Part model, mm, in its own coordinate system. A direction names the side the tool comes from. Round coordinates to 2 decimals unless told otherwise and drop trailing zeros. Order: outer loops, then holes, each group sorted by start corner. A loop starts at its lowest first (then second) coordinate and runs counter-clockwise, first axis right, second up. Notation, with made-up numbers: (-26.75, 14.5) - (-9.75, 14.5) arc R25 ccw to (-9.75, 49.5) - close; hole circle Ø4 at (11, -10). An arc over 180 degrees is marked (long way). Return JSON: item names as keys, results as strings. Group by question number.
Item 1: Two-plate mould, pull along Y, no slides. Class faces 4 (the face through (1.174, -2.072, 4.472)), 5 (the face through (-2.381, 0, 4)), 6 (the face through (-0.61, 4.66, 3.14)), 7 (the face through (-3, -2, 0)): released by +Y, released by -Y, zero draft, split by the parting line, or undercut.
Item 2: Drop flat-ended pins along their axis: pin 1 (3 mm diameter, centred on x = 2, y = -3.5, fed in from -Z); pin 2 (5 mm diameter, centred on x = 0, z = -4, fed in from +Y); pin 3 (3 mm diameter, centred on y = -1.5, z = -9, fed in from +X). Give the stop position or say it passes through.
Item 3: Probe probe 1 along Z at (x, y) = (-1.75, 3.25); probe 2 along X at (y, z) = (0.25, 4); probe 3 along Z at (x, y) = (-0.5, 2). List the from-to ranges inside material, lowest first.
Item 4: Saw through at A-A on z = -8. List the corners of the cut face in (x, y).
Item 5: Tool access for faces 1 (the face through (-1.174, 2.072, 4.472)), 2 (the face through (0, 0, -19.05)), 3 (the face through (0.67, -3.04, -9)): list every direction of +Z, -Z, +X, -X, +Y, -Y with a clear straight run to the whole face (end or side of a thin tool).
```python
from build123d import *

# Parameters (mm, degrees)
SKETCH1_W      = 4.699
SKETCH1_H      = 6.35
SKETCH2_R      = 3.1115
EXTRUDE1_DEPTH = 19.05
EXTRUDE2_DEPTH = 3.81
CHAMFER1_SIZE2 = 0.793750001
CHAMFER1_SIZE  = 0.793749999
FILLET1_R      = 0.381
FILLET2_R      = 0.381


with BuildPart() as part:
    # Sketch1 → Revolve1 (revolve)
    with BuildSketch(Plane(origin=(0, 0, 0), x_dir=(1, 0, 0), z_dir=(0, 1, 0))):
        with Locations((2.3495, -3.175)):
            Rectangle(SKETCH1_W, SKETCH1_H)
    revolve(axis=Axis((0, 0, 0), (0, 0, 1)))

    # Sketch2 → Extrude1 (add)
    with BuildSketch(Plane(origin=(0, 0, 0), x_dir=(-1, 0, 0), z_dir=(0, 0, -1))):
        Circle(SKETCH2_R)
    extrude(amount=EXTRUDE1_DEPTH)

    # Sketch3 → Extrude2 (cut)
    with BuildSketch(Plane.XY.offset(6.35)):
        Polygon((2.38125, 1.374815329), (0, 2.749630657), (-2.38125, 1.374815329), (-2.38125, -1.374815329), (0, -2.749630657), (2.38125, -1.374815329), align=None)
    extrude(amount=-EXTRUDE2_DEPTH, mode=Mode.SUBTRACT)

    # Chamfer1
    chamfer1_edges = [part.edges().sort_by_distance(p)[0] for p in [
        (3.1115, 0, -19.05),
    ]]
    chamfer(chamfer1_edges, length=CHAMFER1_SIZE, length2=CHAMFER1_SIZE2)

    # Fillet1
    fillet1_edges = [part.edges().sort_by_distance(p)[0] for p in [
        (-4.699, 0, 6.35),
    ]]
    fillet(fillet1_edges, radius=FILLET1_R)

    # Fillet2
    fillet2_edges = [part.edges().sort_by_distance(p)[0] for p in [
        (-4.699, 0, 0),
    ]]
    fillet(fillet2_edges, radius=FILLET2_R)


solid = part.part
```
Filled in:
{
 "1": {"face 4": "undercut", "face 5": "undercut", "face 6": "split by the parting line", "face 7": "zero draft"},
 "2": {"pin 1": "stops at z = -18.84", "pin 2": "stops at y = 3.11", "pin 3": "stops at x = 3.11"},
 "3": {"probe 1": "z = 0 to 6.35", "probe 2": "x = -4.69 to -2.38, 2.38 to 4.69", "probe 3": "z = -19.05 to 2.54"},
 "4": {"outline": "circle Ø6.22 at (0, 0)"},
 "5": {"face 1": "+Z", "face 2": "-Z, +X, -X, +Y, -Y", "face 3": "-Z"}
}
